Autodesk Inventor part; units mm, degrees
ref_plane "YZ Plane" through (0, 0, 0) normal (1, 0, 0) x (0, 1, 0)
ref_plane "XZ Plane" through (0, 0, 0) normal (0, 1, 0) x (-1, 0, 0)
ref_plane "XY Plane" through (0, 0, 0) normal (0, 0, 1) x (1, 0, 0)
sketch "Sketch1" plane through (0, 0, 0) normal (0, 0, 1) x (1, 0, 0)
  circle A0 centre (0, 0) radius 55
  dimension "d0" = 110
extrude "Extrusion1" add sketch "Sketch1" along normal blind 1.5
sketch "Sketch2" plane through (0, 0, 1.5) normal (0, 0, 1) x (1, 0, 0)
  circle A0 centre (0, 0) radius 52
  dimension "d3" = 104
extrude "Extrusion2" add sketch "Sketch2" along normal blind 2.5
sketch "Sketch4" plane through (0, 0, 4) normal (0, 0, 1) x (1, 0, 0)
  point P0 (0, 0)
  point P1 (0, 0)
hole "Hole1" at (0, 0, 4) direction (0, 0, -1) diameter 6.6 end through all
sketch "Sketch5" plane through (0, 0, 0) normal (0, 0, -1) x (-1, 0, 0)
  circle A0 centre (0, 0) radius 15 construction
  point P0 (15, 0)
  point P1 (0, -15)
  point P2 (-15, 0)
  point P3 (0, 15)
  dimension "d13" = 30
hole "Hole2" at (-15, 0, 0) at (0, -15, 0) at (15, 0, 0) at (0, 15, 0) direction (0, 0, 1) diameter 3.4 depth 8 tip angle 118 countersink diameter 6.3 countersink angle 90
properties part number "Seconday_End_Top" material "Polycarbonate, Clear"
Geometry check sheet. Reference: the model listing, model coordinates, mm. A direction names the side the tool comes from. Give positions to 0.01 mm unless a question says otherwise; leave off trailing zeros. Order: outer loops, then holes, each group sorted by start corner. A loop starts at its lowest first (then second) coordinate and runs counter-clockwise, first axis right, second up.
1. Scan lines: line 1 (Y direction, x = 0, z = 0.85); line 2 (Y direction, x = 15, z = 2.55); line 3 (X direction, y = 2, z = 3.55). Record each from-to range of solid material in increasing order.
Completed:
line 1: y = -55 to -17.3, -12.7 to -3.3, 3.3 to 12.7, 17.3 to 55
line 2: y = -49.79 to -1.7, 1.7 to 49.79
line 3: x = -51.96 to -2.62, 2.62 to 51.96
2. Depth check by flat-ended pin: pin 1 (4.5 mm diameter, centred on x = 15, y = 0, fed in from -Z); pin 2 (3 mm diameter, centred on x = 0, y = 15, fed in from -Z). Enter the tip coordinate at first touch or a pass-through.
Completed:
pin 1: stops at z = 0.9
pin 2: passes through
3. Sectioned sample at A-A (y = 0). Record the boundary of the cut face in (x, z).
Completed:
outline: (-55, 0) - (-18.15, 0) - (-16.7, 1.45) - (-16.7, 4) - (-52, 4) - (-52, 1.5) - (-55, 1.5) - close; (-13.3, 1.45) - (-11.85, 0) - (-3.3, 0) - (-3.3, 4) - (-13.3, 4) - close; (3.3, 0) - (11.85, 0) - (13.3, 1.45) - (13.3, 4) - (3.3, 4) - close; (16.7, 1.45) - (18.15, 0) - (55, 0) - (55, 1.5) - (52, 1.5) - (52, 4) - (16.7, 4) - close
4. Sectioned sample at D-D (x = 35.5). Record the boundary of the cut face in (y, z).
Completed:
outline: (-42.01, 0) - (42.01, 0) - (42.01, 1.5) - (38, 1.5) - (38, 4) - (-38, 4) - (-38, 1.5) - (-42.01, 1.5) - close
5. Sectioned sample at B-B (y = 15). Record the boundary of the cut face in (x, z).
Completed:
outline: (-52.92, 0) - (-3.15, 0) - (-1.7, 1.45) - (-1.7, 4) - (-49.79, 4) - (-49.79, 1.5) - (-52.92, 1.5) - close; (1.7, 1.45) - (3.15, 0) - (52.92, 0) - (52.92, 1.5) - (49.79, 1.5) - (49.79, 4) - (1.7, 4) - close
6. Sectioned sample at C-C (z = 2.65). Record the boundary of the cut face in (x, y), then the cut area to 3 significant figures.
Completed:
outline: circle Ø104 at (0, 0); hole circle Ø3.4 at (-15, 0); hole circle Ø6.6 at (0, 0); hole circle Ø3.4 at (0, -15); hole circle Ø3.4 at (0, 15); hole circle Ø3.4 at (15, 0)
area: 8,420 mm2
7. Draft check along X on faces 1 (the face through (-41.265, 31.641, 2.732)), 2 (the face through (11, 1, 4)), 3 (the face through (-2.23, 2.43, 1.97)). Enter one of: pulls with the +X half, pulls with the -X half, needs draft (parallel to the pull), parting line crosses it, or undercut.
Completed:
face 1: parting line crosses it
face 2: needs draft
face 3: undercut
8. Access from +Z, -Z, +X, -X, +Y, -Y to the whole of each face (thin tool, end or side, straight path). Record for faces 4 (the face through (20, -49, 1.5)), 5 (the face through (-1, -11, 0)).
Completed:
face 4: +Z
face 5: -Z, +X, -X, +Y, -Y
